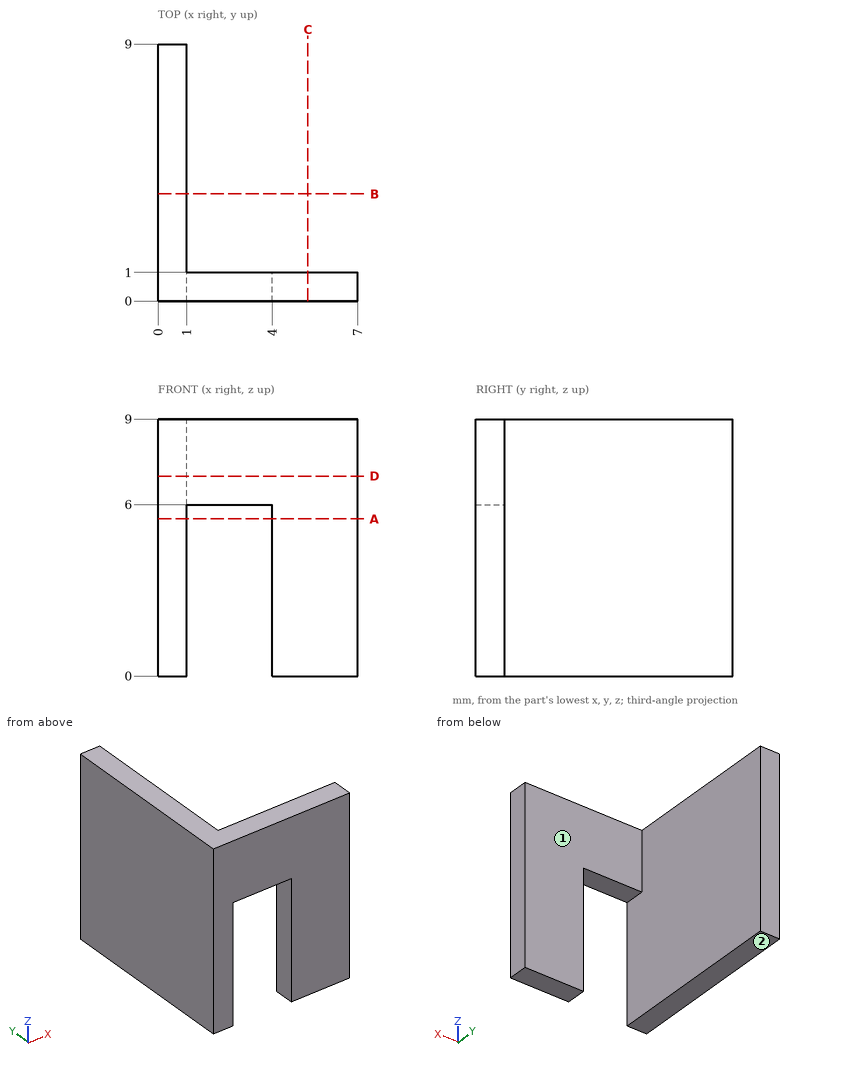
For this review, use the dimensioned drawing (mm, ordinates from the lowest corner) and the shaded views. A direction names the side the tool comes from. Round coordinates to 2 decimals unless told otherwise and drop trailing zeros. Order: outer loops, then holes, each group sorted by start corner. A loop starts at its lowest first (then second) coordinate and runs counter-clockwise, first axis right, second up.
1) Clearance check with flat-ended pins moving along their axes: pin 1 Ø2.5 at (y, z) = (4.5, 5) entering from +X; pin 2 Ø1 at (x, z) = (5.5, 5) entering from +Y; pin 3 Ø1.1 at (x, y) = (2.5, 0.5) entering from -Z. State where each tip first meets the part, or that it passes through.
The answers:
pin 1: stops at x = 1
pin 2: stops at y = 1
pin 3: stops at z = 6
2) Machinability: for the marked faces 1 and 2, which of the approach directions +Z, -Z, +X, -X, +Y, -Y give a long, thin tool a straight path to every point of the face, cutting with its end or side? Answer none if there is none.
The answers:
face 1: +Z, -Z, +X, +Y
face 2: -Z, +X, -X, +Y, -Y
3) Consider section A-A (z = 5.5). State the section outline as (x, y) points, plus the area to 3 significant figures.
The answers:
outline: (0, 0) - (1, 0) - (1, 9) - (0, 9) - close; (4, 0) - (7, 0) - (7, 1) - (4, 1) - close
area: 12.0 mm2
4) Consider section B-B (y = 3.75). State the section outline as (x, z) points.
The answers:
outline: (0, 0) - (1, 0) - (1, 9) - (0, 9) - close
5) For L1, parallel to X at y = 2, z = 5, list the stretches that pass through material, from the lowest coordinate up.
The answers:
L1: x = 0 to 1
6) Consider section D-D (z = 7). State the section outline as (x, y) points.
The answers:
outline: (0, 0) - (7, 0) - (7, 1) - (1, 1) - (1, 9) - (0, 9) - close
